from build123d import *

# Parameters (mm, degrees)
BOSS_EXTRUDE1_DEPTH = 51
SKETCH2_R           = 1
CUT_EXTRUDE1_DEPTH  = 789


with BuildPart() as part:
    # Sketch1 → Boss-Extrude1 (new body)
    with BuildSketch(Plane(origin=(0, 0, 0), x_dir=(0, 0, -1), z_dir=(1, 0, 0))):
        with BuildLine():
            Line((12.15786554, -12.350689419), (15.15786554, -12.350689419))
            Line((15.15786554, -12.350689419), (15.15786554, -7.350689419))
            Line((15.15786554, -7.350689419), (19.19786554, -7.350689419))
            Line((19.19786554, -7.350689419), (19.19786554, -4.350689419))
            Line((19.19786554, -4.350689419), (13.110953215, -4.350689419))
            ThreePointArc((13.110953215, -4.350689419), (1.498781312, -1.097418994), (-6.796190756, -9.850689419))
            Line((-6.796190756, -9.850689419), (-9.80213446, -9.850689419))
            Line((-9.80213446, -9.850689419), (-9.80213446, -12.350689419))
            Line((-9.80213446, -12.350689419), (-2.94213446, -12.350689419))
            ThreePointArc((-2.94213446, -12.350689419), (4.60786554, -4.800689419), (12.15786554, -12.350689419))
        make_face()
    extrude(amount=BOSS_EXTRUDE1_DEPTH)

    # Sketch2 → Cut-Extrude1 (cut)
    with BuildSketch(Plane(origin=(0, -4.350689419, 0), x_dir=(1, 0, 0), z_dir=(0, 1, 0))):
        with Locations((10, 17.19786554)):
            Circle(SKETCH2_R)
        with Locations((41, 17.19786554)):
            Circle(SKETCH2_R)
    extrude(amount=-CUT_EXTRUDE1_DEPTH, mode=Mode.SUBTRACT)


solid = part.part
Geometry check sheet. Reference: the model listing, model coordinates, mm. A direction names the side the tool comes from. Round coordinates to 2 decimals unless told otherwise and drop trailing zeros. Write each loop counter-clockwise with the first axis right and the second up, starting at its lowest first coordinate (ties: lowest second). Pieces come first, ordered by that corner, then holes.
Item 1: Access from +Z, -Z, +X, -X, +Y, -Y to the whole of each face (thin tool, end or side, straight path). Record for faces 1 (the face through (25, -12.351, 6)), 2 (the face through (25, -10, -15.158)), 3 (the face through (25, -4.351, -16)).
Determined:
face 1: +Z, -Z, +X, -X, -Y
face 2: -Z, +X, -X, -Y
face 3: -Z, +X, -X, +Y
Item 2: Material ranges on line 1 along Z through (x, y) = (41, -5.4); line 2 along Z through (x, y) = (10, -6.55); line 3 along Z through (x, y) = (22.5, -11), recorded low to high.
Determined:
line 1: z = -19.2 to -18.2, -16.2 to -7.56, -1.66 to 4.77
line 2: z = -19.2 to -18.2, -16.2 to -9.44, 0.22 to 5.52
line 3: z = -15.16 to -12.04, 2.82 to 9.8
Item 3: Section check B-B (z = -6). Record the boundary of the cut face in (x, y), plus the area to 3 significant figures.
Determined:
outline: (0, -4.93) - (51, -4.93) - (51, -0.76) - (0, -0.76) - close
area: 213 mm2
Item 4: Section check A-A (x = 10). Record the boundary of the cut face in (y, z).
Determined:
outline: (-12.35, -15.16) - (-7.35, -15.16) - (-7.35, -16.2) - (-4.35, -16.2) - (-4.35, -13.11) arc R11.67 ccw to (-9.85, 6.8) - (-9.85, 9.8) - (-12.35, 9.8) - (-12.35, 2.94) arc R7.55 cw to (-12.35, -12.16) - close; (-7.35, -19.2) - (-4.35, -19.2) - (-4.35, -18.2) - (-7.35, -18.2) - close
Item 5: Go/stop test with flat-tipped pins: pin 1 Ø3 at (y, z) = (-7, -2.5) entering from +X; pin 2 Ø2.5 at (x, z) = (10, -17.2) entering from -Y; pin 3 Ø2.5 at (x, z) = (41, -17.2) entering from +Y; pin 4 Ø1.5 at (x, y) = (31.5, -9.5) entering from -Z. Record where each tip stops, or that it passes through.
Determined:
pin 1: passes through
pin 2: stops at y = -7.35
pin 3: stops at y = -4.35
pin 4: stops at z = -15.16
Item 6: Mould release check, pull along X, two halves, no side actions. Record for faces 4 (the face through (9.26, -5.83, -17.87)), 5 (the face through (51, -4, -4)), 6 (the face through (25, -9.851, 8)): +X half, -X half, draft (parallel to the pull), parting line (faces both ways), or undercut.
Determined:
face 4: undercut
face 5: +X half
face 6: draft
Item 7: Section check C-C (y = -1.5). Record the boundary of the cut face in (x, z), plus the area to 3 significant figures.
Determined:
outline: (0, -8.92) - (51, -8.92) - (51, -0.3) - (0, -0.3) - close
area: 439 mm2
